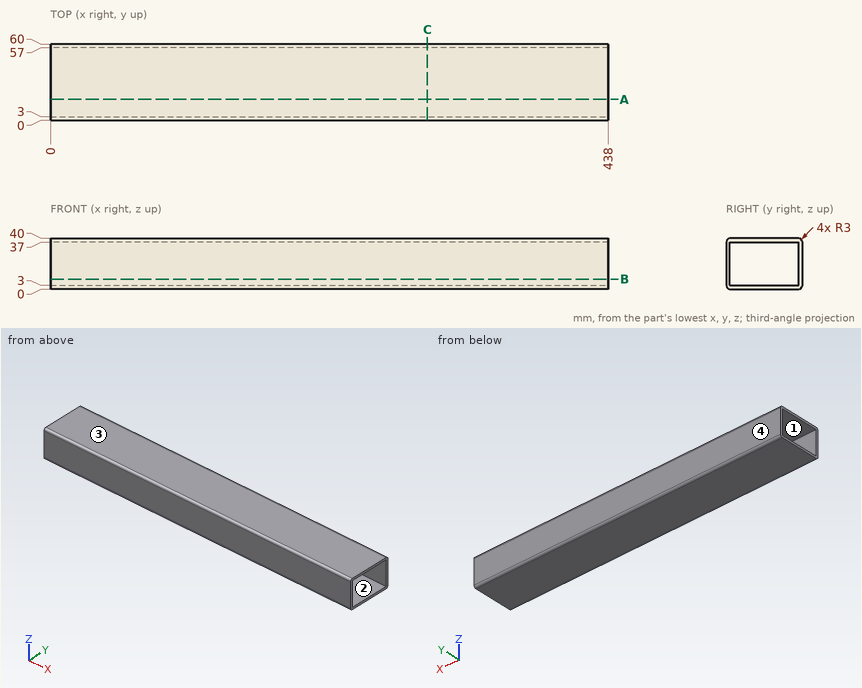
Could you check a few things on this drawing? It's one solid part, dimensions in mm from its lowest x, y, z. Round coordinates to 2 decimals unless told otherwise and drop trailing zeros. Order: outer loops, then holes, each group sorted by start corner. A loop starts at its lowest first (then second) coordinate and runs counter-clockwise, first axis right, second up. Notation, with made-up numbers: M 0,-29 L 58,-29 A14 cw 58,-10 Z; hole C -38.5,-2.75 d7. An arc over 180 degrees is marked long. Return JSON: item names as keys, results as strings. Group by question number.
1. If we section it at C-C on x = 296: List the corners of the cut face in (y, z) for me, then the cut area to 3 significant figures.
2. If we section it at A-A on y = 16.5: List the corners of the cut face in (x, z) for me.
3. Please list where these lines run through material, in increasing order: probe 1 along Z at (x, y) = (30, 21.5); probe 2 along Y at (x, z) = (371, 9); probe 3 along Y at (x, z) = (168, 38).
4. I'm going to push a flat-ended pin straight in: pin 1 Ø8 at (x, z) = (250.5, 35) entering from -Y. Where does the tip first touch, or does it pass through?
5. If we section it at B-B on z = 8: List the corners of the cut face in (x, y) for me.
6. If we mould it in two halves opening along Y, with no side actions, what happens to the marked faces 1, 2, 3 and 4? For each: pulls with the +Y half, pulls with the -Y half, needs draft (parallel to the pull), parting line crosses it, or undercut.
Reply:
{
 "1": {"outline": "M 0,3 A3 ccw 3,0 L 57,0 A3 ccw 60,3 L 60,37 A3 ccw 57,40 L 3,40 A3 ccw 0,37 Z; hole M 3,3 L 57,3 L 57,37 L 3,37 Z", "area": "556 mm^2"},
 "2": {"outline": "M 0,0 L 438,0 L 438,3 L 0,3 Z; M 0,37 L 438,37 L 438,40 L 0,40 Z"},
 "3": {"probe 1": "0 to 3, 37 to 40", "probe 2": "0 to 3, 57 to 60", "probe 3": "0.17 to 59.83"},
 "4": {"pin 1": "y = 0"},
 "5": {"outline": "M 0,0 L 438,0 L 438,3 L 0,3 Z; M 0,57 L 438,57 L 438,60 L 0,60 Z"},
 "6": {"face 1": "undercut", "face 2": "undercut", "face 3": "needs draft", "face 4": "pulls with the +Y half"}
}
